Autodesk Inventor part; units mm, degrees
ref_plane "YZ Plane" through (0, 0, 0) normal (1, 0, 0) x (0, 1, 0)
ref_plane "XZ Plane" through (0, 0, 0) normal (0, 1, 0) x (-1, 0, 0)
ref_plane "XY Plane" through (0, 0, 0) normal (0, 0, 1) x (1, 0, 0)
sketch "Sketch1" plane through (0, 0, 0) normal (1, 0, 0) x (0, 1, 0)
  line L0 (0, 0) -> (-114.3, 0)
  line L1 (-114.3, 0) -> (-114.3, -114.3)
  line L2 (-114.3, -114.3) -> (0, -114.3)
  line L3 (0, -114.3) -> (0, 0)
  dimension "d0" = 114.3
  dimension "d1" = 114.3
extrude "Extrusion1" add sketch "Sketch1" along normal blind 76.2
sketch "Sketch2" plane through (76.2, 0, 0) normal (1, 0, 0) x (0, 0, -1)
  circle A0 centre (30, -30) radius 10
  circle A1 centre (84.3, -30) radius 10
  line L0 (25.4, -68.9) -> (88.9, -68.9)
  line L1 (88.9, -68.9) -> (88.9, -88.9)
  line L2 (88.9, -88.9) -> (25.4, -88.9)
  line L3 (25.4, -88.9) -> (25.4, -68.9)
  line L4 (114.3, 0) -> (0, 0)
  line L5 (114.3, -114.3) -> (114.3, 0)
  line L6 (0, 0) -> (0, -114.3)
  line L7 (0, -114.3) -> (114.3, -114.3)
  dimension "d4" = 20
  dimension "d5" = 20
  dimension "d6" = 63.5
  dimension "d7" = 20
  dimension "d8" = 30
  dimension "d9" = 30
  dimension "d10" = 30
  dimension "d11" = 30
  dimension "d12" = 25.4
  dimension "d13" = 25.4
extrude "Extrusion2" cut sketch "Sketch2" against normal through all contours A0 | A1 | L0 L1 L2 L3
sketch "Sketch3" plane through (76.2, 0, 0) normal (1, 0, 0) x (0, 0, -1)
  point P0 (0, 0)
fillet "Fillet2" radius 8 4 edges at (76.2, -57.15, 0) (76.2, 0, -57.15) (76.2, -114.3, -57.15) (76.2, -57.15, -114.3)
sketch "Sketch4" plane through (76.2, 0, 0) normal (1, 0, 0) x (0, 0, -1)
  point P0 (0, 0)
sketch "Sketch5" plane through (0, 0, 0) normal (-1, 0, 0) x (0, 0, 1)
  circle A0 centre (-57.15, -25.4) radius 2
  circle A1 centre (-57.15, -101.6) radius 2
  line L0 (-114.3, 0) -> (0, 0)
  line L1 (0, -114.3) -> (-114.3, -114.3)
  line L2 (-114.3, -114.3) -> (-114.3, 0)
  dimension "d18" = 4
  dimension "d19" = 4
  dimension "d20" = 25.4
  dimension "d21" = 12.7
  dimension "d22" = 57.15
  dimension "d23" = 57.15
extrude "Extrusion3" cut sketch "Sketch5" against normal blind 25.4
properties part number "face" material "PBT Plastic"
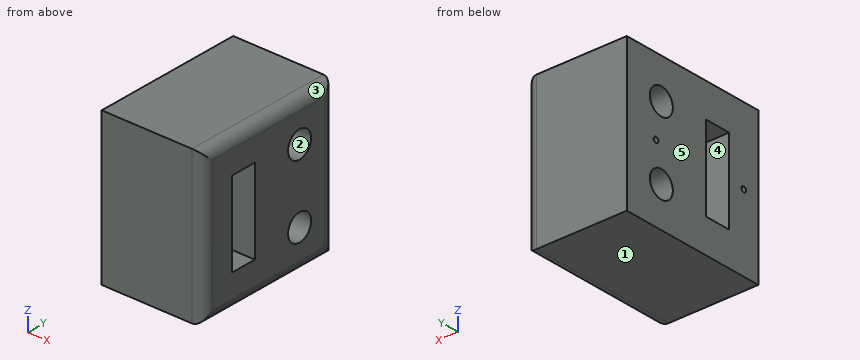
Here's how the part is built. I have some questions about the finished solid (model axes, mm). Face numbers are marked on the shaded views. A direction names the side the tool comes from. Give positions to 0.01 mm unless a question says otherwise; leave off trailing zeros. Order: outer loops, then holes, each group sorted by start corner. A loop starts at its lowest first (then second) coordinate and runs counter-clockwise, first axis right, second up. Notation, with made-up numbers: (29.5, 47) -> (60.5, 47) arc R10 ccw to (60.5, 54) -> close; hole circle Ø10 at (51, 25). An arc over 180 degrees is marked (long way). Use a Markdown table: item, result. Add a question column.
Item 1: Imagine slicing it at C-C on x = 14. Please give me the cut outline in (y, z), plus the area to 3 significant figures.
Item 2: Imagine slicing it at B-B on y = -30. Please give me the cut outline in (x, z).
Item 3: I need wall thicknesses on line 1 (Y direction, x = 42.5, z = -84.3); line 2 (Y direction, x = 10.75, z = -57.15); line 3 (Y direction, x = 4.5, z = -50.5). Which ranges of each line are inside material? Lowest first, please.
Item 4: If we mould it in two halves opening along Z, with no side actions, what happens to the marked faces 1, 2 and 3? For each: pulls with the +Z half, pulls with the -Z half, needs draft (parallel to the pull), parting line crosses it, or undercut.
Item 5: For the marked faces 4 and 5, which set-ups out of +Z, -Z, +X, -X, +Y, -Y let a thin tool reach every point of the face, with its end or its side?
Item 6: Imagine slicing it at D-D on z = -84.3. Please give me the cut outline in (x, y), plus the area to 3 significant figures.
Item 7: Will these pins go through, and if not, where does the flat tip stop? pin 1 (2 mm diameter, centred on y = -101.5, z = -58, fed in from -X); pin 2 (16 mm diameter, centred on y = -30, z = -30, fed in from +X).
Item 8: Imagine slicing it at A-A on z = -57.15. Please give me the cut outline in (x, y).
Data:
| question | item | result |
|---|---|---|
| 1 | outline | (-114.3, -114.3) -> (0, -114.3) -> (0, 0) -> (-114.3, 0) -> close; hole circle Ø4 at (-101.6, -57.15); hole (-88.9, -88.9) -> (-68.9, -88.9) -> (-68.9, -25.4) -> (-88.9, -25.4) -> close; hole circle Ø20 at (-30, -84.3); hole circle Ø20 at (-30, -30); hole circle Ø4 at (-25.4, -57.15) |
| 1 | area | 11,100 mm² |
| 2 | outline | (0, -114.3) -> (68.2, -114.3) arc R8 ccw to (76.2, -106.3) -> (76.2, -94.3) -> (0, -94.3) -> close; (0, -74.3) -> (76.2, -74.3) -> (76.2, -40) -> (0, -40) -> close; (0, -20) -> (76.2, -20) -> (76.2, -8) arc R8 ccw to (68.2, 0) -> (0, 0) -> close |
| 3 | line 1 | y = -114.3 to -88.9, -68.9 to -40, -20 to 0 |
| 3 | line 2 | y = -114.3 to -103.6, -99.6 to -88.9, -68.9 to -27.4, -23.4 to 0 |
| 3 | line 3 | y = -114.3 to -88.9, -68.9 to 0 |
| 4 | face 1 | pulls with the -Z half |
| 4 | face 2 | undercut |
| 4 | face 3 | pulls with the +Z half |
| 5 | face 4 | +X, -X |
| 5 | face 5 | +Z, -Z, -X, +Y, -Y |
| 6 | outline | (0, -114.3) -> (68.2, -114.3) arc R8 ccw to (76.2, -106.3) -> (76.2, -88.9) -> (0, -88.9) -> close; (0, -68.9) -> (76.2, -68.9) -> (76.2, -40) -> (0, -40) -> close; (0, -20) -> (76.2, -20) -> (76.2, -8) arc R8 ccw to (68.2, 0) -> (0, 0) -> close |
| 6 | area | 5,630 mm² |
| 7 | pin 1 | stops at x = 25.4 |
| 7 | pin 2 | passes through |
| 8 | outline | (0, -114.3) -> (68.2, -114.3) arc R8 ccw to (76.2, -106.3) -> (76.2, -88.9) -> (0, -88.9) -> (0, -99.6) -> (25.4, -99.6) -> (25.4, -103.6) -> (0, -103.6) -> close; (0, -68.9) -> (76.2, -68.9) -> (76.2, -8) arc R8 ccw to (68.2, 0) -> (0, 0) -> (0, -23.4) -> (25.4, -23.4) -> (25.4, -27.4) -> (0, -27.4) -> close |
